Design review of the part built by this model. Coordinates are the model's own, in mm. A direction names the side the tool comes from. Coordinates: 2 decimals unless noted, no trailing zeros. Loops run counter-clockwise (first coordinate to the right, second up) from the corner with the lowest first, then second, coordinate; pieces in that order, holes last. Notation, with made-up numbers: (-7.5, 4.5) -> (49.5, 4.5) arc R5 cw to (49.5, 11.5) -> close; hole circle Ø6 at (59, -6). An arc over 180 degrees is marked (long way). Use one line per item in the form item = value. Start each with the question number.
1. Consider section B-B (z = 0.5). State the section outline as (x, y) points (3 decimals).
2. Machinability: for faces 1 (the face through (41.275, -1, 4)), 2 (the face through (46, -25.4, 42)), 3 (the face through (32.65, 12.52, 51.53)), 4 (the face through (22.225, -21, 18)), which of the approach directions +Z, -Z, +X, -X, +Y, -Y give a long, thin tool a straight path to every point of the face, cutting with its end or side? Answer none if there is none.
3. Wall thickness on line 1 (X direction, y = -19, z = 11) (3 decimals); line 2 (X direction, y = 43, z = -0.5) (3 decimals); line 3 (Y direction, x = 69.5, z = 55): over which ranges is each line inside the solid? List them lowest first. Write a range as from..to.
4. Consider section C-C (y = 33). State the section outline as (x, z) points (3 decimals).
5. Consider section A-A (y = -18.5). State the section outline as (x, z) points (3 decimals).
6. For pin 1 (1.5 mm diameter, centred on x = 31.5, y = 9, fed in from +Z); pin 2 (14 mm diameter, centred on x = 69.5, y = 7.5, fed in from -Z); pin 3 (15.5 mm diameter, centred on x = 52, z = 26.5, fed in from -Y); pin 4 (24 mm diameter, centred on x = -16.5, y = -45.5, fed in from +Z) (3 decimals), all flat-tipped, find the tip position at first contact; note any pin that passes through.
from build123d import *

# Parameters (mm, degrees)
F1_DEPTH = 63.5
F2_DEPTH = 15.875
F3_DEPTH = 25.4


with BuildPart() as f1:
    # F0 (on Front) → F1 (new body, symmetric)
    with BuildSketch(Plane.XZ):
        Polygon((-41.275, 9.525), (-41.275, -9.525), (41.275, -9.525), (41.275, 9.525), (22.225, 9.525), align=None)
    extrude(amount=F1_DEPTH, both=True)

    # F0 (on Front) → F2 (join)
    with BuildSketch(Plane.XZ):
        with BuildLine():
            add(Edge.make_bspline(
                [(-41.275, 9.525), (-40.5575186014, 45.8087362349), (13.0318803713, 61.4552721381), (57.0519533598, 61.9252)],
                knots=[0, 0, 0, 0, 111.4179999689, 111.4179999689, 111.4179999689, 111.4179999689], degree=3))
            Line((-41.275, 9.525), (22.225, 9.525))
            Line((22.225, 9.525), (22.225, 26.3727564465))
            ThreePointArc((22.225, 26.3727564465), (32.3824338056, 51.2569528518), (57.0519533598, 61.9252))
        make_face()
    extrude(amount=F2_DEPTH)

    # F0 (on Front) → F3 (join, symmetric)
    with BuildSketch(Plane.XZ):
        with BuildLine():
            Line((22.225, 9.525), (41.275, 9.525))
            Line((41.275, 9.525), (41.275, 26.3727564465))
            ThreePointArc((41.275, 26.3727564465), (45.935398186, 37.8691487872), (57.2855435312, 42.8752))
            Line((57.2855435312, 42.8752), (59.8077454329, 42.8752))
            Line((59.8077454329, 42.8752), (59.8077454329, 61.9252))
            Line((59.8077454329, 61.9252), (57.0519533598, 61.9252))
            ThreePointArc((57.0519533598, 61.9252), (32.3824338056, 51.2569528518), (22.225, 26.3727564465))
            Line((22.225, 26.3727564465), (22.225, 9.525))
        make_face()
        Polygon((85.0275978446, 61.9252), (59.8077454329, 61.9252), (59.8077454329, 42.8752), (85.327843825, 42.8752), (85.2077454329, 52.4002), align=None)
    extrude(amount=F3_DEPTH, both=True)


solid = f1.part
Geometry check:
q1.outline = (-41.275, -63.5) -> (41.275, -63.5) -> (41.275, 63.5) -> (-41.275, 63.5) -> close
q2.face_1 = -Z, +X, +Y, -Y
q2.face_2 = +Z, +X, -X, -Y
q2.face_3 = +Z, -X, +Y
q2.face_4 = +Z, -X, -Y
q3.line_1 = 22.225..41.275
q3.line_2 = -41.275..41.275
q3.line_3 = -25.4..25.4
q4.outline = (-41.275, -9.525) -> (41.275, -9.525) -> (41.275, 9.525) -> (-41.275, 9.525) -> close
q5.outline = (-41.275, -9.525) -> (41.275, -9.525) -> (41.275, 26.373) arc R16.51 cw to (57.286, 42.875) -> (85.328, 42.875) -> (85.208, 52.4) -> (85.028, 61.925) -> (57.052, 61.925) arc R35.56 ccw to (22.225, 26.373) -> (22.225, 9.525) -> (-41.275, 9.525) -> close
q6.pin_1 = 51.12
q6.pin_2 = 42.88
q6.pin_3 = through
q6.pin_4 = 9.525
